Verification items for the finished model (mm, model axes). A direction names the side the tool comes from. Give positions to 0.01 mm unless a question says otherwise; leave off trailing zeros. Loops run counter-clockwise (first coordinate to the right, second up) from the corner with the lowest first, then second, coordinate; pieces in that order, holes last. Notation, with made-up numbers: (39, 50.5) - (98, 50.5) arc R32 cw to (98, 81.5) - close; hole circle Ø5 at (52.25, -12). An arc over 180 degrees is marked (long way). Answer in a Markdown table with one row per item.
```python
from build123d import *

# Parameters (mm, degrees)
F3_W     = 8.1543137785
F3_H     = 2
F5_DEPTH = 9
F6_DEPTH = 6
F8_R     = 2


# Not quite as in the source:
# - a feature names something its author has since deleted; it is built from what else it names


with BuildPart() as f4:
    # F3 (on Front) → F4 (revolve)
    with BuildSketch(Plane.XZ):
        with Locations((6.3856310444, -2.5)):
            Rectangle(F3_W, F3_H)
    revolve(axis=Axis((6.3856310444, 0, -1.5), (1, 0, 0)))

    # F3 (on Front) → F5 (join, symmetric)
    with BuildSketch(Plane.XZ):
        with BuildLine():
            ThreePointArc((-9, 1), (-7.232233047, 0.267766953), (-6.5, -1.5))
            Line((-6.5, -1.5), (-3.5, -1.5))
            Line((-3.5, -1.5), (-3.5, 4))
            Line((-3.5, 4), (-9, 4))
            Line((-9, 4), (-9, 1))
        make_face()
        with BuildLine():
            Line((-3.5, -1.5), (-6.5, -1.5))
            ThreePointArc((-6.5, -1.5), (-7.232233047, -3.267766953), (-9, -4))
            Line((-9, -4), (-9, -7))
            Line((-9, -7), (-3.5, -7))
            Line((-3.5, -7), (-3.5, -1.5))
        make_face()
        with BuildLine():
            Line((-9, -7), (-9, -4))
            ThreePointArc((-9, -4), (-10.767766953, -3.267766953), (-11.5, -1.5))
            Line((-11.5, -1.5), (-14.5, -1.5))
            Line((-14.5, -1.5), (-14.5, -7))
            Line((-14.5, -7), (-9, -7))
        make_face()
        with BuildLine():
            ThreePointArc((-11.5, -1.5), (-10.767766953, 0.267766953), (-9, 1))
            Line((-9, 1), (-9, 4))
            Line((-9, 4), (-14.5, 4))
            Line((-14.5, 4), (-14.5, -1.5))
            Line((-14.5, -1.5), (-11.5, -1.5))
        make_face()
        Polygon((0, 1.8910123945), (0, -1.5), (2.3084741551, -1.5), (2.3084741551, 0.5), align=None)
        Polygon((2.3084741551, -1.5), (0, -1.5), (0, -4.8910123945), (2.3084741551, -3.5), align=None)
        Polygon((-3.5, 4), (-3.5, -1.5), (0, -1.5), (0, 1.8910123945), align=None)
        Polygon((0, -1.5), (-3.5, -1.5), (-3.5, -7), (0, -4.8910123945), align=None)
    extrude(amount=F5_DEPTH, both=True)


with BuildPart() as f6:
    # F3 (on Front) → F6 (new body, symmetric)
    with BuildSketch(Plane.XZ):
        with BuildLine():
            ThreePointArc((-11.5, -1.5), (-10.767766953, 0.267766953), (-9, 1))
            Line((-9, 1), (-9, 4))
            Line((-9, 4), (-14.5, 4))
            Line((-14.5, 4), (-14.5, -1.5))
            Line((-14.5, -1.5), (-11.5, -1.5))
        make_face()
        with BuildLine():
            ThreePointArc((-9, 1), (-7.232233047, 0.267766953), (-6.5, -1.5))
            Line((-6.5, -1.5), (-3.5, -1.5))
            Line((-3.5, -1.5), (-3.5, 4))
            Line((-3.5, 4), (-9, 4))
            Line((-9, 4), (-9, 1))
        make_face()
        with BuildLine():
            Line((-3.5, -1.5), (-6.5, -1.5))
            ThreePointArc((-6.5, -1.5), (-7.232233047, -3.267766953), (-9, -4))
            Line((-9, -4), (-9, -7))
            Line((-9, -7), (-3.5, -7))
            Line((-3.5, -7), (-3.5, -1.5))
        make_face()
        with BuildLine():
            Line((-9, -7), (-9, -4))
            ThreePointArc((-9, -4), (-10.767766953, -3.267766953), (-11.5, -1.5))
            Line((-11.5, -1.5), (-14.5, -1.5))
            Line((-14.5, -1.5), (-14.5, -7))
            Line((-14.5, -7), (-9, -7))
        make_face()
        Polygon((-3.5, 4), (-3.5, -1.5), (0, -1.5), (0, 1.8910123945), align=None)
        Polygon((0, -1.5), (-3.5, -1.5), (-3.5, -7), (0, -4.8910123945), align=None)
    extrude(amount=F6_DEPTH, both=True)


with BuildPart() as f4_1:
    add(f4.part)

    # F7: cut F6
    add(f6.part, mode=Mode.SUBTRACT)

    # F8
    f8_edges = [f4_1.edges().sort_by_distance(p)[0] for p in [
        (-9, -9, 4),
        (-9, -9, -7),
        (-9, 9, -7),
        (-9, 9, 4),
    ]]
    fillet(f8_edges, radius=F8_R)


solid = f4_1.part
```
Q1. Go/stop test with flat-tipped pins: P1, Ø2, axis at x = 0, y = -3.5, coming from the -Z side; P2, Ø1.2, axis at y = -6.5, z = -1, coming from the +X side; P3, Ø1.5, axis at x = 6.5, z = -4.5, coming from the +Y side. Record where each tip stops, or that it passes through.
Completed:
| item | result |
|---|---|
| P1 | z = -4.89 |
| P2 | x = 2.31 |
| P3 | through |
Q2. Thickness scan on line 1 (Y direction, x = -5, z = -2.25); line 2 (Z direction, x = -8, y = -7.5); line 3 (Y direction, x = -6, z = 2.75). Record the ranges inside material, lowest first.
Completed:
| item | result |
|---|---|
| line 1 | -9 to -6, 6 to 9 |
| line 2 | -6.94 to -3.79, 0.79 to 3.94 |
| line 3 | -8.85 to -6, 6 to 8.85 |
Q3. Tool access check on faces 1 (the face through (-6, -9, -1)), 2 (the face through (-6, 6, -1)). Record the directions out of +Z, -Z, +X, -X, +Y, -Y that give a thin tool (end or side, any length) a straight path to the whole face; none if there is none.
Completed:
| item | result |
|---|---|
| face 1 | +Z, -Z, +X, -X, -Y |
| face 2 | +Z, -Z, -X |
Q4. Sectioned sample at C-C (z = -2). Record the cut outline in (x, y).
Completed:
| item | result |
|---|---|
| outline | (-14.5, -9) - (-11.45, -9) - (-11.45, -6) - (-14.5, -6) - close; (-14.5, 6) - (-11.45, 6) - (-11.45, 9) - (-14.5, 9) - close; (-6.55, -9) - (2.31, -9) - (2.31, -1.94) - (10.46, -1.94) - (10.46, 1.94) - (2.31, 1.94) - (2.31, 9) - (-6.55, 9) - (-6.55, 6) - (0, 6) - (0, -6) - (-6.55, -6) - close |
Q5. Sectioned sample at B-B (x = -0.75). Record the cut outline in (y, z), and give its area (3 significant figures).
Completed:
| item | result |
|---|---|
| outline | (-9, -5) arc R2 ccw to (-8.97, -5.34) - (-6, -5.34) - (-6, 2.34) - (-8.97, 2.34) arc R2 ccw to (-9, 2) - close; (6, -5.34) - (8.97, -5.34) arc R2 ccw to (9, -5) - (9, 2) arc R2 ccw to (8.97, 2.34) - (6, 2.34) - close |
| area | 46.1 mm^2 |
Q6. Sectioned sample at A-A (z = -6). Record the cut outline in (x, y), and give its area (3 significant figures).
Completed:
| item | result |
|---|---|
| outline | (-14.5, -8.73) - (-1.84, -8.73) - (-1.84, -6) - (-14.5, -6) - close; (-14.5, 6) - (-1.84, 6) - (-1.84, 8.73) - (-14.5, 8.73) - close |
| area | 69.2 mm^2 |
Q7. Sectioned sample at D-D (y = -0.75). Record the cut outline in (x, z).
Completed:
| item | result |
|---|---|
| outline | (0, -4.89) - (2.31, -3.5) - (2.31, -3.35) - (10.46, -3.35) - (10.46, 0.35) - (2.31, 0.35) - (2.31, 0.5) - (0, 1.89) - close |
Q8. Draft check along Y on faces 3 (the face through (-6, -6, -1)), 4 (the face through (10.463, 0, -1)), 5 (the face through (-8.83, 8.43, -6.4)). Enter one of: +Y half, -Y half, draft (parallel to the pull), parting line (faces both ways), or undercut.
Completed:
| item | result |
|---|---|
| face 3 | undercut |
| face 4 | draft |
| face 5 | +Y half |
